Here's how the part is built. I have some questions about the finished solid (model axes, mm). A direction names the side the tool comes from. Coordinates: 2 decimals unless noted, no trailing zeros. Write each loop counter-clockwise with the first axis right and the second up, starting at its lowest first coordinate (ties: lowest second). Pieces come first, ordered by that corner, then holes. Notation, with made-up numbers: (-34.75, 45.25) -> (13.25, 45.25) arc R24 cw to (13.25, 61.25) -> close; hole circle Ø4 at (-23, -27). An arc over 180 degrees is marked (long way). Use CSV: the item, a comma, the result in double quotes. Start each with the question number.
```python
from build123d import *

# Parameters (mm, degrees)
SKETCH_1_W          = 16
SKETCH_1_H          = 6
EXTRUDE_1_DEPTH     = 2
SKETCH_1_3_W        = 16
SKETCH_1_3_H        = 2
SKETCH_1_3_H_2      = 1.5
EXTRUDE_2_DEPTH     = 15
SKETCH_2_W          = 8
SKETCH_2_H          = 26
CUT_EXTRUDE_1_DEPTH = 2
EXTRUDE_3_DEPTH     = 2.5
EXTRUDE_4_DEPTH     = 5
EXTRUDE_5_DEPTH     = 1.5
SKETCH_9_W          = 1.2
SKETCH_9_H          = 1.820432063
EXTRUDE_6_DEPTH     = 2
EXTRUDE_7_DEPTH     = 12
CUT_EXTRUDE_START   = -7.10494
CUT_EXTRUDE_2_DEPTH = 7.10494
SKETCH_12_R         = 1.281793471
CUT_EXTRUDE_3_DEPTH = 10
CUT_EXTRUDE_4_DEPTH = 20.2


with BuildPart() as part:
    # 草图1 → 凸台-拉伸1 (new body)
    with BuildSketch(Plane(origin=(0, 0, 0), x_dir=(1, 0, 0), z_dir=(0, 1, 0))):
        with Locations((0, -0.25)):
            Rectangle(SKETCH_1_W, SKETCH_1_H)
    extrude(amount=EXTRUDE_1_DEPTH)

    # 草图1<3> → 凸台-拉伸2 (add)
    with BuildSketch(Plane(origin=(0, 0, 0), x_dir=(1, 0, 0), z_dir=(0, 1, 0))):
        with Locations((0, 3.75)):
            Rectangle(SKETCH_1_3_W, SKETCH_1_3_H)
        with Locations((0, -4)):
            Rectangle(SKETCH_1_3_W, SKETCH_1_3_H_2)
    extrude(amount=EXTRUDE_2_DEPTH)

    # 草图2 → 切除-拉伸1 (cut)
    with BuildSketch(Plane(origin=(0, 0, -4.75), x_dir=(-1, 0, 0), z_dir=(0, 0, -1))):
        with Locations((0, 15)):
            Rectangle(SKETCH_2_W, SKETCH_2_H)
    extrude(amount=-CUT_EXTRUDE_1_DEPTH, mode=Mode.SUBTRACT)

    # 草图3 → 凸台-拉伸3 (add, symmetric)
    with BuildSketch(Plane(origin=(0, 0, 0), x_dir=(0, 0, -1), z_dir=(1, 0, 0))):
        Polygon((4.75, 0), (8.831597644, 0), (11.768525918, 13.935665169), (4.75, 15.414812878), align=None)
    extrude(amount=EXTRUDE_3_DEPTH, both=True)

    # 草图5 → 凸台-拉伸4 (add)
    with BuildSketch(Plane(origin=(2.5, 0, 0), x_dir=(0, 0, -1), z_dir=(1, 0, 0))):
        Polygon((4.75, 6.451105389), (3.822798244, 8.744995241), (3.822798244, 15.463750373), (4.75, 15.414812878), align=None)
    extrude(amount=-EXTRUDE_4_DEPTH)

    # 草图6 → 凸台-拉伸5 (add)
    with BuildSketch(Plane.ZY.offset(2.5)):
        Polygon((-4.75, 6.451105389), (-10.094945569, 5.994560313), (-11.768525918, 13.935665169), (-4.75, 15.414812878), (-3.822798244, 15.463750373), (-3.822798244, 8.744995241), align=None)
    extrude_5 = extrude(amount=EXTRUDE_5_DEPTH)

    # 草图9 → 凸台-拉伸6 (add)
    with BuildSketch(Plane.XZ):
        with Locations((8.6, -2.660216032)):
            Rectangle(SKETCH_9_W, SKETCH_9_H)
        with Locations((-8.6, -2.660216032)):
            Rectangle(SKETCH_9_W, SKETCH_9_H)
    extrude(amount=-EXTRUDE_6_DEPTH)

    # 草图9<3> → 凸台-拉伸7 (add)
    with BuildSketch(Plane.XZ):
        Polygon((8, -3.570432063), (8, -4.75), (11.2, -4.75), (11.2, -1.75), (9.2, -1.75), (9.2, -3.570432063), align=None)
        Polygon((-8, -4.75), (-8, -3.570432063), (-9.2, -3.570432063), (-9.2, -1.75), (-11.2, -1.75), (-11.2, -4.75), align=None)
    extrude(amount=-EXTRUDE_7_DEPTH)

    # 草图11 → 切除-拉伸2 (cut)
    with BuildSketch(Plane(origin=(0, -1.782098659, -8.456022034), x_dir=(-1, 0, 0), z_dir=(0, -0.206219179, -0.978505825)).offset(CUT_EXTRUDE_START)):
        Polygon((2.5, 7.947483572), (4, 11.245323919), (4, 7.947483572), (4, 5.815044055), (2.5, 5.815044055), align=None)
    cut_extrude_2 = extrude(amount=CUT_EXTRUDE_2_DEPTH, mode=Mode.SUBTRACT)

    # 镜向1: 凸台-拉伸5, 切除-拉伸2 across plane
    add(extrude_5.mirror(Plane(origin=(0, 0, 0), x_dir=(0, 0, 1), z_dir=(1, 0, 0))))
    add(cut_extrude_2.mirror(Plane(origin=(0, 0, 0), x_dir=(0, 0, 1), z_dir=(1, 0, 0))), mode=Mode.SUBTRACT)

    # 草图12 → 切除-拉伸3 (cut)
    with BuildSketch(Plane(origin=(4, 0, 0), x_dir=(0, 0, -1), z_dir=(1, 0, 0))):
        with Locations((9.183579002, 11.7521089)):
            Circle(SKETCH_12_R)
    extrude(amount=-CUT_EXTRUDE_3_DEPTH, mode=Mode.SUBTRACT)

    # 草图13 → 切除-拉伸4 (cut, through all)
    with BuildSketch(Plane(origin=(8, 0, 0), x_dir=(0, 0, -1), z_dir=(1, 0, 0))):
        Polygon((-3.25, 9.484512334), (-4.55, 9.484512334), (-4.55, 0), (-4.75, 0), (-4.75, 15), (-3.25, 15), align=None)
    extrude(amount=-CUT_EXTRUDE_4_DEPTH, mode=Mode.SUBTRACT)


solid = part.part
```
Item 1: If I drill on line 1 along Z through (x, y) = (7.5, 2.5); line 2 along X through (y, z) = (11.75, -10.5); line 3 along Z through (x, y) = (2.75, 3), over which ranges is the centre line in solid material (lowest first)?
Item 2: I want a section at C-C on x = -1.75. Please give me the cut outline in (y, z) (3 decimals).
Item 3: Thinking about a two-plate mould opening in X: for faces 1 (the flat face through (-6, 8, -2.75)), 2 (the flat face through (-11.2, 6, -3)), 3 (the flat face through (0, 2, -1)), 4 (the flat face through (-7, 7, -4.75)), which applies, +X half, -X half, draft (parallel to the pull), parting line (faces both ways), or undercut?
Item 4: I want a section at A-A on x = -6.5. Please give me the cut outline in (y, z), then the cut area to 3 significant figures.
Item 5: I'm going to push flat-ended pins straight in: pin 1 (3.5 mm diameter, centred on x = 0, y = 6.5, fed in from -Z); pin 2 (0.9 mm diameter, centred on x = 9, z = -3.5, fed in from +Y); pin 3 (1 mm diameter, centred on x = -9, y = 9, fed in from +Z). Where does each tip first touch, or does it pass through?
Item 6: I want a section at B-B on y = 4.75. Please give me the cut outline in (x, z).
Item 7: I want a section at D-D on z = -8.25. Please give me the cut outline in (x, y).
Item 8: Which directions (+Z, -Z, +X, -X, +Y, -Y) give clear straight access to the entire face, cutting with the end or side of a thin tool? Please do faces 5 (the flat face through (6, 15, -4)), 6 (the flat face through (-3.24, 8.33, -6.91)), 7 (the flat face through (10, 6, -1.75)), 8 (the flat face through (6, 8, -2.75)).
Geometry says:
1,line 1,"-4.75 to -2.75, 3.25 to 4.55"
1,line 2,"-4 to 4"
1,line 3,"3.25 to 4.55"
2,outline,"(0, -8.832) -> (13.936, -11.769) -> (15.415, -4.75) -> (15.464, -3.823) -> (8.745, -3.823) -> (6.451, -4.75) -> (2, -4.75) -> (2, 3.25) -> (9.485, 3.25) -> (9.485, 4.55) -> (0, 4.55) -> close; hole circle Ø2.564 at (11.752, -9.184)"
3,face 1,"undercut"
3,face 2,"-X half"
3,face 3,"undercut"
3,face 4,"draft"
4,outline,"(0, -4.75) -> (15, -4.75) -> (15, -2.75) -> (2, -2.75) -> (2, 3.25) -> (9.48, 3.25) -> (9.48, 4.55) -> (0, 4.55) -> close"
4,area,"54.3 mm2"
5,pin 1,"z = -10.57"
5,pin 2,"y = 12"
5,pin 3,"z = -1.75"
6,outline,"(-11.2, -4.75) -> (-4, -4.75) -> (-4, -2.75) -> (-8, -2.75) -> (-8, -3.57) -> (-9.2, -3.57) -> (-9.2, -1.75) -> (-11.2, -1.75) -> close; (-8, 3.25) -> (8, 3.25) -> (8, 4.55) -> (-8, 4.55) -> close; (-2.5, -9.83) -> (2.5, -9.83) -> (2.5, -4.75) -> (-2.5, -4.75) -> close; (4, -4.75) -> (11.2, -4.75) -> (11.2, -1.75) -> (9.2, -1.75) -> (9.2, -3.57) -> (8, -3.57) -> (8, -2.75) -> (4, -2.75) -> close"
7,outline,"(-4, 9.75) -> (-2.5, 6.38) -> (-2.5, 0) -> (2.5, 0) -> (2.5, 6.38) -> (4, 9.75) -> (4, 10.87) -> (-4, 10.87) -> close; (-4, 12.63) -> (4, 12.63) -> (4, 14.68) -> (-4, 14.68) -> close"
8,face 5,"+Z, -Z, +X, +Y"
8,face 6,"none"
8,face 7,"+Z, +X, +Y, -Y"
8,face 8,"+Y"
